Check sheet for the modelled part. Datum: model origin and axes. Units: mm. Face numbers are marked on the shaded views. A direction names the side the tool comes from. Round coordinates to 2 decimals unless told otherwise and drop trailing zeros. Order: outer loops, then holes, each group sorted by start corner. A loop starts at its lowest first (then second) coordinate and runs counter-clockwise, first axis right, second up. Notation, with made-up numbers: (31.5, 72) -> (85.5, 72) arc R20 ccw to (85.5, 94) -> close; hole circle Ø6 at (27.5, -8). An arc over 180 degrees is marked (long way). Answer in a Markdown table with one row per item.
Autodesk Inventor part; units mm, degrees
ref_plane "YZ Plane" through (0, 0, 0) normal (1, 0, 0) x (0, 1, 0)
ref_plane "XZ Plane" through (0, 0, 0) normal (0, 1, 0) x (-1, 0, 0)
ref_plane "XY Plane" through (0, 0, 0) normal (0, 0, 1) x (1, 0, 0)
sketch "Szkic1" plane through (0, 0, 0) normal (0, 0, 1) x (1, 0, 0)
  line L0 (-37.6373, 46.6232) -> (29.3627, 46.6232)
  line L1 (29.3627, 46.6232) -> (29.3627, -41.3768)
  line L2 (29.3627, -41.3768) -> (-37.6373, -41.3768)
  line L3 (-37.6373, -41.3768) -> (-37.6373, 46.6232)
  point P0 (0, 0)
  point P1 (-33.6373, 42.6232)
  point P2 (25.3627, 42.6232)
  point P3 (25.3627, -37.3768)
  point P4 (-33.6373, -37.3768)
  dimension "d0" = 88
  dimension "d1" = 67
  dimension "d2" = 59
  dimension "d3" = 80
  dimension "d4" = 80
  dimension "d5" = 59
  dimension "d6" = 4
  dimension "d7" = 4
  dimension "d8" = 4
  dimension "d9" = 4
  dimension "d10" = 4
  dimension "d11" = 4
  dimension "d12" = 4
extrude "Wyciągnięcie proste1" add sketch "Szkic1" along normal blind 1.5
hole "Otwór1" at (-33.6373, 42.6232, 0) at (25.3627, 42.6232, 0) at (25.3627, -37.3768, 0) at (-33.6373, -37.3768, 0) direction (0, 0, 1) diameter 3.6 end through all
sketch "Szkic2" plane through (0, 0, 0) normal (0, 0, -1) x (-1, 0, 0)
  line L0 (-18.8627, 21.1232) -> (31.1373, 21.1232)
  line L1 (31.1373, 21.1232) -> (31.1373, -28.8768)
  line L2 (31.1373, -28.8768) -> (-18.8627, -28.8768)
  line L3 (-18.8627, -28.8768) -> (-18.8627, 21.1232)
  circle A0 centre (-25.3627, -37.3768) radius 1.8
  circle A1 centre (33.6373, 42.6232) radius 1.8
  circle A2 centre (-25.3627, 42.6232) radius 1.8
  circle A3 centre (33.6373, -37.3768) radius 1.8
  line L4 (37.6373, 46.6232) -> (-29.3627, 46.6232)
  line L5 (-29.3627, 46.6232) -> (-29.3627, -41.3768)
  line L6 (-29.3627, -41.3768) -> (37.6373, -41.3768)
  line L7 (37.6373, -41.3768) -> (37.6373, 46.6232)
  line L8 (-16.3627, 42.6232) -> (23.6373, 42.6232)
  line L9 (23.6373, 42.6232) -> (23.6373, 27.6232)
  line L10 (23.6373, 27.6232) -> (-16.3627, 27.6232)
  line L11 (-16.3627, 27.6232) -> (-16.3627, 42.6232)
  point P0 (0, 0)
  dimension "d22" = 50
  dimension "d23" = 50
  dimension "d24" = 6.5
  dimension "d25" = 12.5
  dimension "d26" = 40
  dimension "d27" = 15
  dimension "d28" = 13
  dimension "d29" = 4
extrude "Wyciągnięcie proste2" add sketch "Szkic2" along normal blind 25 contours L0 L1 L2 L3
sketch "Szkic3" plane through (0, 0, -25) normal (0, 0, -1) x (-1, 0, 0)
  line L0 (31.1373, 21.1232) -> (-18.8627, 21.1232)
  line L1 (-18.8627, 21.1232) -> (-18.8627, -28.8768)
  line L2 (-18.8627, -28.8768) -> (31.1373, -28.8768)
  line L3 (31.1373, -28.8768) -> (31.1373, 21.1232)
  line L4 (-18.8627, -28.8768) -> (-18.8627, 21.1232)
  line L5 (-18.8627, -27.5268) -> (31.1373, -27.5268)
  line L6 (31.1373, -27.5268) -> (31.1373, -25.1768)
  line L7 (31.1373, -25.1768) -> (-18.8627, -25.1768)
  line L8 (-18.8627, -25.1768) -> (-18.8627, -27.5268)
  line L9 (-18.8627, -23.7768) -> (31.1373, -23.7768)
  line L10 (31.1373, -23.7768) -> (31.1373, -21.4268)
  line L11 (31.1373, -21.4268) -> (-18.8627, -21.4268)
  line L12 (-18.8627, -21.4268) -> (-18.8627, -23.7768)
  line L13 (-18.8627, -20.0268) -> (31.1373, -20.0268)
  line L14 (31.1373, -20.0268) -> (31.1373, -17.6768)
  line L15 (31.1373, -17.6768) -> (-18.8627, -17.6768)
  line L16 (-18.8627, -17.6768) -> (-18.8627, -20.0268)
  line L17 (-18.8627, -16.2768) -> (31.1373, -16.2768)
  line L18 (31.1373, -16.2768) -> (31.1373, -13.9268)
  line L19 (31.1373, -13.9268) -> (-18.8627, -13.9268)
  line L20 (-18.8627, -13.9268) -> (-18.8627, -16.2768)
  line L21 (-18.8627, -12.5268) -> (31.1373, -12.5268)
  line L22 (31.1373, -12.5268) -> (31.1373, -10.1768)
  line L23 (31.1373, -10.1768) -> (-18.8627, -10.1768)
  line L24 (-18.8627, -10.1768) -> (-18.8627, -12.5268)
  line L25 (-18.8627, -8.7768) -> (31.1373, -8.7768)
  line L26 (31.1373, -8.7768) -> (31.1373, -6.4268)
  line L27 (31.1373, -6.4268) -> (-18.8627, -6.4268)
  line L28 (-18.8627, -6.4268) -> (-18.8627, -8.7768)
  line L29 (-18.8627, -5.0268) -> (31.1373, -5.0268)
  line L30 (31.1373, -5.0268) -> (31.1373, -2.6768)
  line L31 (31.1373, -2.6768) -> (-18.8627, -2.6768)
  line L32 (-18.8627, -2.6768) -> (-18.8627, -5.0268)
  line L33 (-18.8627, -1.2768) -> (31.1373, -1.2768)
  line L34 (31.1373, -1.2768) -> (31.1373, 1.0732)
  line L35 (31.1373, 1.0732) -> (-18.8627, 1.0732)
  line L36 (-18.8627, 1.0732) -> (-18.8627, -1.2768)
  line L37 (-18.8627, 2.4732) -> (31.1373, 2.4732)
  line L38 (31.1373, 2.4732) -> (31.1373, 4.8232)
  line L39 (31.1373, 4.8232) -> (-18.8627, 4.8232)
  line L40 (-18.8627, 4.8232) -> (-18.8627, 2.4732)
  line L41 (-18.8627, 6.2232) -> (31.1373, 6.2232)
  line L42 (31.1373, 6.2232) -> (31.1373, 8.5732)
  line L43 (31.1373, 8.5732) -> (-18.8627, 8.5732)
  line L44 (-18.8627, 8.5732) -> (-18.8627, 6.2232)
  line L45 (-18.8627, 9.9732) -> (31.1373, 9.9732)
  line L46 (31.1373, 9.9732) -> (31.1373, 12.3232)
  line L47 (31.1373, 12.3232) -> (-18.8627, 12.3232)
  line L48 (-18.8627, 12.3232) -> (-18.8627, 9.9732)
  line L49 (-18.8627, 13.7232) -> (31.1373, 13.7232)
  line L50 (31.1373, 13.7232) -> (31.1373, 16.0732)
  line L51 (31.1373, 16.0732) -> (-18.8627, 16.0732)
  line L52 (-18.8627, 16.0732) -> (-18.8627, 13.7232)
  line L53 (-18.8627, 17.4732) -> (31.1373, 17.4732)
  line L54 (31.1373, 17.4732) -> (31.1373, 19.8232)
  line L55 (31.1373, 19.8232) -> (-18.8627, 19.8232)
  line L56 (-18.8627, 19.8232) -> (-18.8627, 17.4732)
  point P0 (0, 0)
  dimension "d32" = 50
  dimension "d33" = 2.35
  dimension "d34" = 1.35
  dimension "d37" = 3.75
extrude "Wyciągnięcie proste3" cut sketch "Szkic3" against normal blind 17 contours L3 L53 L1 L55 | L3 L49 L1 L51 | L3 L45 L1 L47 | L3 L41 L1 L43 | L3 L37 L1 L39 | L3 L33 L1 L35 | L3 L29 L1 L31 | L3 L25 L1 L27 | L3 L21 L1 L23 | L3 L17 L1 L19 | L3 L13 L1 L15 | L3 L9 L1 L11 | L3 L5 L1 L7
sketch "Szkic4" plane through (-31.1373, -28.8768, 0) normal (-1, 0, 0) x (0, 0, 1)
  line L0 (-8, 42.6) -> (-25, 42.6)
  line L1 (-25, 41.2) -> (-25, 42.6)
  line L2 (-25, 41.2) -> (-8, 41.2)
  line L3 (-8, 41.2) -> (-8, 38.85)
  line L4 (-8, 38.85) -> (-25, 38.85)
  line L5 (-25, 37.45) -> (-25, 38.85)
  line L6 (-25, 37.45) -> (-8, 37.45)
  line L7 (-8, 37.45) -> (-8, 35.1)
  line L8 (-8, 35.1) -> (-25, 35.1)
  line L9 (-25, 33.7) -> (-25, 35.1)
  line L10 (-25, 33.7) -> (-8, 33.7)
  line L11 (-8, 33.7) -> (-8, 31.35)
  line L12 (-8, 31.35) -> (-25, 31.35)
  line L13 (-25, 29.95) -> (-25, 31.35)
  line L14 (-25, 29.95) -> (-8, 29.95)
  line L15 (-8, 29.95) -> (-8, 27.6)
  line L16 (-8, 27.6) -> (-25, 27.6)
  line L17 (-25, 26.2) -> (-25, 27.6)
  line L18 (-25, 26.2) -> (-8, 26.2)
  line L19 (-8, 26.2) -> (-8, 23.85)
  line L20 (-8, 23.85) -> (-25, 23.85)
  line L21 (-25, 22.45) -> (-25, 23.85)
  line L22 (-25, 22.45) -> (-8, 22.45)
  line L23 (-8, 22.45) -> (-8, 20.1)
  line L24 (-8, 20.1) -> (-25, 20.1)
  line L25 (-25, 18.7) -> (-25, 20.1)
  line L26 (-25, 18.7) -> (-8, 18.7)
  line L27 (-8, 18.7) -> (-8, 16.35)
  line L28 (-8, 16.35) -> (-25, 16.35)
  line L29 (-25, 14.95) -> (-25, 16.35)
  line L30 (-25, 14.95) -> (-8, 14.95)
  line L31 (-8, 14.95) -> (-8, 12.6)
  line L32 (-8, 12.6) -> (-25, 12.6)
  line L33 (-25, 11.2) -> (-25, 12.6)
  line L34 (-25, 11.2) -> (-8, 11.2)
  line L35 (-8, 11.2) -> (-8, 8.85)
  line L36 (-8, 8.85) -> (-25, 8.85)
  line L37 (-25, 7.45) -> (-25, 8.85)
  line L38 (-25, 7.45) -> (-8, 7.45)
  line L39 (-8, 7.45) -> (-8, 5.1)
  line L40 (-8, 5.1) -> (-25, 5.1)
  line L41 (-25, 3.7) -> (-25, 5.1)
  line L42 (-25, 3.7) -> (-8, 3.7)
  line L43 (-8, 3.7) -> (-8, 1.35)
  line L44 (-8, 1.35) -> (-25, 1.35)
  line L45 (-25, 0) -> (-25, 1.35)
  line L46 (0, 0) -> (-25, 0)
  line L47 (0, 50) -> (0, 0)
  line L48 (0, 50) -> (-25, 50)
  line L49 (-25, 48.7) -> (-25, 50)
  line L50 (-25, 48.7) -> (-8, 48.7)
  line L51 (-8, 48.7) -> (-8, 46.35)
  line L52 (-8, 46.35) -> (-25, 46.35)
  line L53 (-25, 44.95) -> (-25, 46.35)
  line L54 (-25, 44.95) -> (-8, 44.95)
  line L55 (-8, 44.95) -> (-8, 42.6)
  line L56 (0, 50) -> (0, 0)
  line L57 (0, 50) -> (-25, 50)
  line L58 (0, 0) -> (-5, 0)
  line L59 (-5, 0) -> (-5, 50)
  line L60 (-5, 50) -> (0, 50)
  line L61 (0, 50) -> (0, 0)
  point P0 (0, 28.8768)
  dimension "d44" = 5
extrude "Wyciągnięcie proste4" cut sketch "Szkic4" against normal blind 16 contours L48 L47 L46 L59
sketch "Szkic5" plane through (18.8627, -28.8768, 0) normal (1, 0, 0) x (0, 0, -1)
  line L0 (25, 42.6) -> (8, 42.6)
  line L1 (8, 42.6) -> (8, 44.95)
  line L2 (8, 44.95) -> (25, 44.95)
  line L3 (25, 46.35) -> (25, 44.95)
  line L4 (25, 46.35) -> (8, 46.35)
  line L5 (8, 46.35) -> (8, 48.7)
  line L6 (8, 48.7) -> (25, 48.7)
  line L7 (25, 50) -> (25, 48.7)
  line L8 (0, 50) -> (25, 50)
  line L9 (0, 0) -> (0, 50)
  line L10 (0, 0) -> (25, 0)
  line L11 (25, 1.35) -> (25, 0)
  line L12 (25, 1.35) -> (8, 1.35)
  line L13 (8, 1.35) -> (8, 3.7)
  line L14 (8, 3.7) -> (25, 3.7)
  line L15 (25, 5.1) -> (25, 3.7)
  line L16 (25, 5.1) -> (8, 5.1)
  line L17 (8, 5.1) -> (8, 7.45)
  line L18 (8, 7.45) -> (25, 7.45)
  line L19 (25, 8.85) -> (25, 7.45)
  line L20 (25, 8.85) -> (8, 8.85)
  line L21 (8, 8.85) -> (8, 11.2)
  line L22 (8, 11.2) -> (25, 11.2)
  line L23 (25, 12.6) -> (25, 11.2)
  line L24 (25, 12.6) -> (8, 12.6)
  line L25 (8, 12.6) -> (8, 14.95)
  line L26 (8, 14.95) -> (25, 14.95)
  line L27 (25, 16.35) -> (25, 14.95)
  line L28 (25, 16.35) -> (8, 16.35)
  line L29 (8, 16.35) -> (8, 18.7)
  line L30 (8, 18.7) -> (25, 18.7)
  line L31 (25, 20.1) -> (25, 18.7)
  line L32 (25, 20.1) -> (8, 20.1)
  line L33 (8, 20.1) -> (8, 22.45)
  line L34 (8, 22.45) -> (25, 22.45)
  line L35 (25, 23.85) -> (25, 22.45)
  line L36 (25, 23.85) -> (8, 23.85)
  line L37 (8, 23.85) -> (8, 26.2)
  line L38 (8, 26.2) -> (25, 26.2)
  line L39 (25, 27.6) -> (25, 26.2)
  line L40 (25, 27.6) -> (8, 27.6)
  line L41 (8, 27.6) -> (8, 29.95)
  line L42 (8, 29.95) -> (25, 29.95)
  line L43 (25, 31.35) -> (25, 29.95)
  line L44 (25, 31.35) -> (8, 31.35)
  line L45 (8, 31.35) -> (8, 33.7)
  line L46 (8, 33.7) -> (25, 33.7)
  line L47 (25, 35.1) -> (25, 33.7)
  line L48 (25, 35.1) -> (8, 35.1)
  line L49 (8, 35.1) -> (8, 37.45)
  line L50 (8, 37.45) -> (25, 37.45)
  line L51 (25, 38.85) -> (25, 37.45)
  line L52 (25, 38.85) -> (8, 38.85)
  line L53 (8, 38.85) -> (8, 41.2)
  line L54 (8, 41.2) -> (25, 41.2)
  line L55 (25, 42.6) -> (25, 41.2)
  line L56 (5, 0) -> (5, 50)
  point P0 (0, 28.8768)
extrude "Wyciągnięcie proste5" cut sketch "Szkic5" against normal blind 16 contours L56 L10 L9 L8
sketch "Szkic6" plane through (-31.1373, 21.1232, -25) normal (0, 1, 0) x (1, 0, 0)
  line L0 (34, -25) -> (34, -20)
  line L1 (34, -20) -> (50, -20)
  line L2 (50, -20) -> (50, 0)
  line L3 (0, 0) -> (50, 0)
  line L4 (0, -20) -> (0, 0)
  line L5 (0, -20) -> (16, -20)
  line L6 (16, -20) -> (16, -25)
  line L7 (34, -25) -> (16, -25)
  line L8 (16, -25) -> (16, -20)
  line L9 (34, -20) -> (50, -20)
  line L10 (16, -25) -> (34, -25)
  line L11 (34, -25) -> (34, -20)
  line L12 (34, -20) -> (16, -20)
  line L13 (16, -20) -> (16, -25)
  point P0 (31.1373, -25)
extrude "Wyciągnięcie proste6" cut sketch "Szkic6" against normal blind 12 contours L7 L6 L12 L0
sketch "Szkic7" plane through (-31.1373, -28.8768, -25) normal (0, -1, 0) x (1, 0, 0)
  line L0 (34, 20) -> (34, 25)
  line L1 (16, 25) -> (34, 25)
  line L2 (16, 25) -> (16, 20)
  line L3 (16, 20) -> (0, 20)
  line L4 (0, 20) -> (0, 0)
  line L5 (50, 0) -> (0, 0)
  line L6 (50, 20) -> (50, 0)
  line L7 (50, 20) -> (34, 20)
  line L8 (16, 20) -> (34, 20)
  point P0 (31.1373, 25)
extrude "Wyciągnięcie proste7" cut sketch "Szkic7" against normal blind 12 contours L8 L2 L1 L0
extrude "Wyciągnięcie proste8" add sketch "Szkic2" along normal blind 4.5 contours L8 L9 L10 L11
sketch "Szkic8" plane through (0, 0, -4.5) normal (0, 0, -1) x (-1, 0, 0)
  line L0 (23.6373, 42.6232) -> (-16.3627, 42.6232)
  line L1 (-16.3627, 42.6232) -> (-16.3627, 27.6232)
  line L2 (-16.3627, 27.6232) -> (23.6373, 27.6232)
  line L3 (23.6373, 27.6232) -> (23.6373, 42.6232)
  line L4 (-16.3627, 27.6232) -> (23.6373, 27.6232)
  line L5 (23.6373, 27.6232) -> (23.6373, 46.1232)
  line L6 (23.6373, 46.1232) -> (-16.3627, 46.1232)
  line L7 (-16.3627, 46.1232) -> (-16.3627, 27.6232)
  point P0 (0, 0)
  dimension "d55" = 40
  dimension "d56" = 18.5
extrude "Wyciągnięcie proste9" add sketch "Szkic8" along normal blind 13
sketch "Szkic9" plane through (0, 0, -17.5) normal (0, 0, -1) x (-1, 0, 0)
  line L0 (-16.3627, 27.6232) -> (23.6373, 27.6232)
  line L1 (23.6373, 27.6232) -> (23.6373, 46.1232)
  line L2 (23.6373, 46.1232) -> (-16.3627, 46.1232)
  line L3 (-16.3627, 46.1232) -> (-16.3627, 27.6232)
  line L4 (23.6373, 42.6232) -> (-16.3627, 42.6232)
  point P0 (0, 0)
extrude "Wyciągnięcie proste10" add sketch "Szkic9" along normal blind 12 contours L3 L4 L1 L0
sketch "Szkic10" plane through (0, 0, -29.5) normal (0, 0, -1) x (-1, 0, 0)
  line L0 (-16.3627, 27.6232) -> (23.6373, 27.6232)
  line L1 (23.6373, 27.6232) -> (23.6373, 42.6232)
  line L2 (23.6373, 42.6232) -> (-16.3627, 42.6232)
  line L3 (-16.3627, 42.6232) -> (-16.3627, 27.6232)
  point P0 (0, 0)
  point P1 (18.7191, 35.1232)
  point P2 (8.7191, 35.1232)
  point P3 (-1.2809, 35.1232)
  point P4 (-11.2809, 35.1232)
  dimension "d61" = 15
  dimension "d62" = 7.5
  dimension "d63" = 7.5
  dimension "d64" = 7.5
  dimension "d65" = 7.5
  dimension "d66" = 10
  dimension "d67" = 10
  dimension "d68" = 10
hole "Otwór2" at (-18.7191, 35.1232, -29.5) at (-8.7191, 35.1232, -29.5) at (1.2809, 35.1232, -29.5) at (11.2809, 35.1232, -29.5) direction (0, 0, 1) diameter 6.4 depth 3.6
properties part number "COTS_Generic_MKS_Mosfet_Module_For_Heatbed"
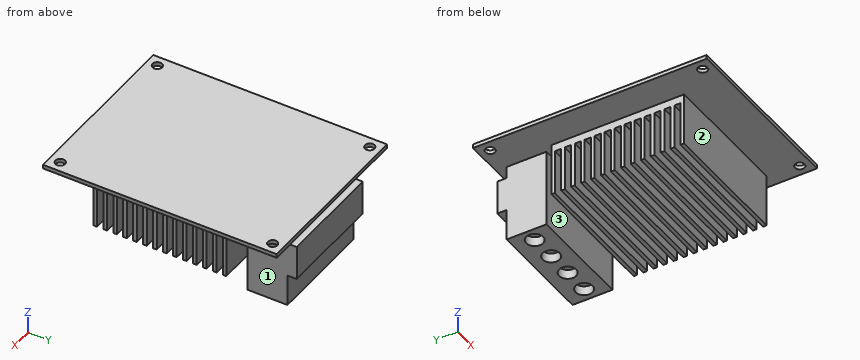
Item 1: Depth check by flat-ended pin: P1, Ø2, axis at x = -21.5, z = -9, coming from the +Y side; P2, Ø5, axis at x = -8.5, y = 34.5, coming from the -Z side; P3, Ø4, axis at x = -15.5, y = -25.5, coming from the -Z side; P4, Ø1, axis at y = -29.5, z = -15, coming from the -X side. Enter the tip coordinate at first touch or a pass-through.
Result sheet:
| item | result |
|---|---|
| P1 | stops at y = 46.12 |
| P2 | stops at z = -25.9 |
| P3 | stops at z = -25 |
| P4 | passes through |
Item 2: Cross-section at A-A (z = -3.5). Record the boundary of the cut face in (x, y), and give its area (3 significant figures).
Result sheet:
| item | result |
|---|---|
| outline | (-23.64, 27.62) -> (16.36, 27.62) -> (16.36, 42.62) -> (-23.64, 42.62) -> close; (-15.14, -16.88) -> (2.86, -16.88) -> (2.86, 9.12) -> (-15.14, 9.12) -> close |
| area | 1,070 mm^2 |
Item 3: Cross-section at C-C (z = -13). State how many separate pieces and enclosed holes the cut face has, and give its area (3 significant figures).
Result sheet:
| item | result |
|---|---|
| separate pieces | 15 |
| enclosed holes | 0 |
| area | 1,710 mm^2 |
Item 4: Set-up check for the marked faces 1, 2 and 3: record each of +Z, -Z, +X, -X, +Y, -Y from which the full face is reachable in a straight line by a thin tool's end or side.
Result sheet:
| item | result |
|---|---|
| face 1 | -Z, +X, +Y |
| face 2 | -Z, +X, -X, -Y |
| face 3 | -Z, +X, -X |
Item 5: Cross-section at B-B (y = 3.5). Record the boundary of the cut face in (x, z).
Result sheet:
| item | result |
|---|---|
| outline | (-37.64, 0) -> (-15.14, 0) -> (-15.14, -5) -> (-31.14, -5) -> (-31.14, -8) -> (18.86, -8) -> (18.86, -5) -> (2.86, -5) -> (2.86, 0) -> (29.36, 0) -> (29.36, 1.5) -> (-37.64, 1.5) -> close |
Item 6: Scan lines: line 1 (Z direction, x = -23, y = -18); line 2 (Z direction, x = 16.5, y = -24); line 3 (Y direction, x = -8.5, z = -4). Record each from-to range of solid material in increasing order. Write a range as [from, to].
Result sheet:
| item | result |
|---|---|
| line 1 | z = [-8, -5], [0, 1.5] |
| line 2 | z = [-25, -5], [0, 1.5] |
| line 3 | y = [-16.88, 9.12], [27.62, 42.62] |
Item 7: Cross-section at D-D (x = 20). Record the boundary of the cut face in (y, z), and give its area (3 significant figures).
Result sheet:
| item | result |
|---|---|
| outline | (-41.38, 0) -> (46.62, 0) -> (46.62, 1.5) -> (-41.38, 1.5) -> close |
| area | 132 mm^2 |
